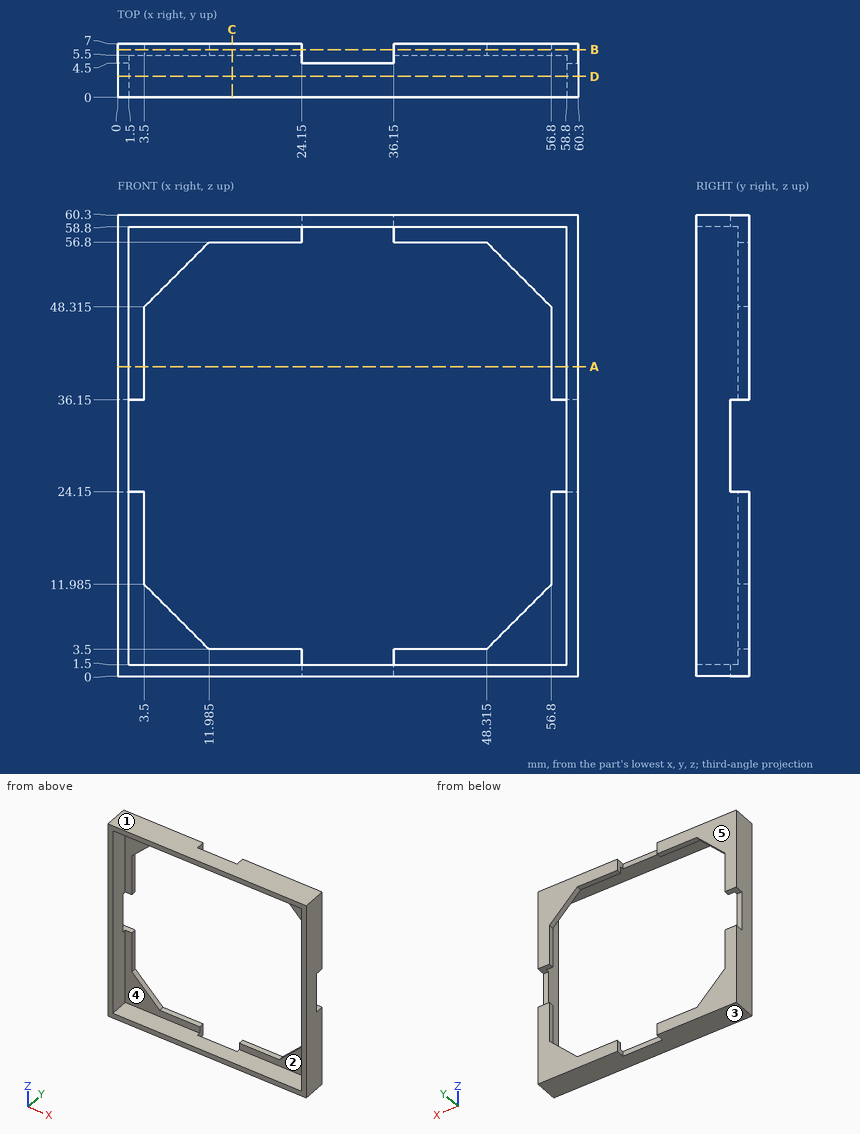
Can you work these out from the drawing? Everything is in mm from the part's minimum corner. A direction names the side the tool comes from. Round coordinates to 2 decimals unless told otherwise and drop trailing zeros. Order: outer loops, then holes, each group sorted by start corner. A loop starts at its lowest first (then second) coordinate and runs counter-clockwise, first axis right, second up. Notation, with made-up numbers: (-15.5, -22) -> (3.5, -22) arc R23 cw to (3.5, 4) -> close; hole circle Ø11 at (44, 26). An arc over 180 degrees is marked (long way). Return JSON: item names as keys, results as strings. Group by question number.
1. If we section it at D-D, the plane y = 2.75: Write out the boundary of the cut face in (x, z).
2. If we section it at C-C, the plane x = 15: Write out the boundary of the cut face in (y, z), then the cut area to 3 significant figures.
3. I need wall thicknesses on line 1 (X direction, y = 6.75, z = 44.5); line 2 (Z direction, x = 41.5, y = 3.5). Which ranges of each line are inside material? Lowest first, please. Write a range as [from, to].
4. Will these pins go through, and if not, where does the flat tip stop? pin 1 (1.2 mm diameter, centred on x = 31, z = 0.5, fed in from +Y); pin 2 (18 mm diameter, centred on x = 47, z = 11.5, fed in from -Y).
5. Which directions (+Z, -Z, +X, -X, +Y, -Y) give clear straight access to the entire face, cutting with the end or side of a thin tool? Please do the marked faces 1 and 2.
6. If we section it at A-A, the plane z = 40.5: Write out the boundary of the cut face in (x, y).
7. If we section it at B-B, the plane y = 6.25: Count the separate pieces of the cut face and the enclosed holes in it, then the cut area to 3 significant figures.
8. We'd pull the mould along Z, two halves only. Please class the marked faces 3, 4 and 5: released by +Z, released by -Z, zero draft, split by the parting line, or undercut.
Output values:
{
 "1": {"outline": "(0, 0) -> (60.3, 0) -> (60.3, 60.3) -> (0, 60.3) -> close; hole (1.5, 1.5) -> (58.8, 1.5) -> (58.8, 58.8) -> (1.5, 58.8) -> close"},
 "2": {"outline": "(0, 0) -> (7, 0) -> (7, 3.5) -> (5.5, 3.5) -> (5.5, 1.5) -> (0, 1.5) -> close; (0, 58.8) -> (5.5, 58.8) -> (5.5, 56.8) -> (7, 56.8) -> (7, 60.3) -> (0, 60.3) -> close", "area": "27.0 mm²"},
 "3": {"line 1": "[0, 3.5], [56.8, 60.3]", "line 2": "[0, 1.5], [58.8, 60.3]"},
 "4": {"pin 1": "y = 4.5", "pin 2": "y = 5.5"},
 "5": {"face 1": "+Z, +X, -X, +Y, -Y", "face 2": "-Y"},
 "6": {"outline": "(0, 0) -> (1.5, 0) -> (1.5, 5.5) -> (3.5, 5.5) -> (3.5, 7) -> (0, 7) -> close; (56.8, 5.5) -> (58.8, 5.5) -> (58.8, 0) -> (60.3, 0) -> (60.3, 7) -> (56.8, 7) -> close"},
 "7": {"separate pieces": "4", "enclosed holes": "0", "area": "771 mm²"},
 "8": {"face 3": "released by -Z", "face 4": "undercut", "face 5": "zero draft"}
}
